```python
from build123d import *

# Parameters (mm, degrees)
SKETCH_1_W          = 1980
SKETCH_1_H          = 530
SKETCH_1_W_2        = 1920
SKETCH_1_H_2        = 470
EXTRUDE_1_DEPTH     = 30
SKETCH_2_W          = 68
SKETCH_2_H          = 30
EXTRUDE_2_DEPTH     = 68
SKETCH_3_R          = 23.5
CUT_EXTRUDE_1_DEPTH = 1125.999555555
SKETCH_4_W          = 31
SKETCH_4_H          = 470
EXTRUDE_3_DEPTH     = 30
SKETCH_5_R          = 3
CUT_EXTRUDE_2_DEPTH = 1030.528532873
SKETCH_6_R          = 3
CUT_EXTRUDE_3_DEPTH = 1030.528532873
SKETCH_7_W          = 883.399544852
SKETCH_7_H          = 30
CUT_EXTRUDE_4_DEPTH = 1125.999555555
SKETCH_8_R          = 3
CUT_EXTRUDE_5_DEPTH = 1125.999555555


with BuildPart() as part:
    # 草图1 → 凸台-拉伸1 (new body)
    with BuildSketch(Plane(origin=(0, 0, 0), x_dir=(1, 0, 0), z_dir=(0, 1, 0))):
        Rectangle(SKETCH_1_W, SKETCH_1_H)
        Rectangle(SKETCH_1_W_2, SKETCH_1_H_2, mode=Mode.SUBTRACT)
    extrude(amount=EXTRUDE_1_DEPTH)

    # 草图2 → 凸台-拉伸2 (add)
    with BuildSketch(Plane.XZ):
        with Locations((0, 250)):
            Rectangle(SKETCH_2_W, SKETCH_2_H)
        with Locations((0, -250)):
            Rectangle(SKETCH_2_W, SKETCH_2_H)
    extrude(amount=EXTRUDE_2_DEPTH)

    # 草图3 → 切除-拉伸1 (cut, through all)
    with BuildSketch(Plane.XY.offset(265)):
        with Locations((0, -30)):
            Circle(SKETCH_3_R)
    extrude(amount=-CUT_EXTRUDE_1_DEPTH, mode=Mode.SUBTRACT)

    # 草图4 → 凸台-拉伸3 (add)
    with BuildSketch(Plane(origin=(0, 30, 0), x_dir=(1, 0, 0), z_dir=(0, 1, 0))):
        with Locations((764.5, 0)):
            Rectangle(SKETCH_4_W, SKETCH_4_H)
    extrude(amount=-EXTRUDE_3_DEPTH)

    # 草图5 → 切除-拉伸2 (cut, through all)
    with BuildSketch(Plane(origin=(0, 30, 0), x_dir=(1, 0, 0), z_dir=(0, 1, 0))):
        with Locations(Location((759, 180, 0), (0, 0, 270))):
            Circle(SKETCH_5_R)
        with Locations(Location((774.5, 180, 0), (0, 0, 270))):
            Circle(SKETCH_5_R)
        with Locations(Location((759, -180, 0), (0, 0, 270))):
            Circle(SKETCH_5_R)
        with Locations(Location((774.5, -180, 0), (0, 0, 270))):
            Circle(SKETCH_5_R)
    extrude(amount=-CUT_EXTRUDE_2_DEPTH, mode=Mode.SUBTRACT)

    # 草图6 → 切除-拉伸3 (cut, symmetric)
    with BuildSketch(Plane(origin=(0, 30, 0), x_dir=(1, 0, 0), z_dir=(0, 1, 0))):
        with Locations(Location((840, -250, 0), (0, 0, 270))):
            Circle(SKETCH_6_R)
    cut_extrude_3 = extrude(amount=CUT_EXTRUDE_3_DEPTH, both=True, mode=Mode.SUBTRACT)

    # 镜向1: 切除-拉伸3 across plane
    add(cut_extrude_3.mirror(Plane.XY), mode=Mode.SUBTRACT)

    # 草图7 → 切除-拉伸4 (cut, through all)
    with BuildSketch(Plane.XY.offset(265)):
        with Locations((-591.699772426, 15)):
            Rectangle(SKETCH_7_W, SKETCH_7_H)
    extrude(amount=-CUT_EXTRUDE_4_DEPTH, mode=Mode.SUBTRACT)

    # 草图8 → 切除-拉伸5 (cut, through all)
    with BuildSketch(Plane.XY.offset(265)):
        with Locations((-100, 15)):
            Circle(SKETCH_8_R)
    extrude(amount=-CUT_EXTRUDE_5_DEPTH, mode=Mode.SUBTRACT)


solid = part.part
```
Read the model definition and answer for the solid it produces. Units are mm, in the model's axes. A direction names the side the tool comes from. Coordinates: 2 decimals unless noted, no trailing zeros. Loops run counter-clockwise (first coordinate to the right, second up) from the corner with the lowest first, then second, coordinate; pieces in that order, holes last.
(1) The mould has two halves that part along Z. Classify faces 1 (the face through (-93, 0, -250)), 2 (the face through (960, 15, 3)): released by +Z, released by -Z, zero draft, split by the parting line, or undercut.
Solution:
face 1: zero draft
face 2: undercut
(2) The part is cut by section A-A (y = -30). Determine the outline of the cut face in (x, z).
Solution:
outline: (-34, -265) - (-23.5, -265) - (-23.5, -235) - (-34, -235) - close; (-34, 235) - (-23.5, 235) - (-23.5, 265) - (-34, 265) - close; (23.5, -265) - (34, -265) - (34, -235) - (23.5, -235) - close; (23.5, 235) - (34, 235) - (34, 265) - (23.5, 265) - close
(3) Flat-ended cylindrical pins translate along their axes: pin 1 Ø24 at (y, z) = (-42.5, 249.5) entering from -X; pin 2 Ø15 at (y, z) = (15, 107.5) entering from -X; pin 3 Ø9 at (y, z) = (-43.5, -256.5) entering from +X. Find the tip coordinate at first contact, or state that the pin passes through.
Solution:
pin 1: stops at x = -34
pin 2: stops at x = 749
pin 3: stops at x = 34
(4) The part is cut by section C-C (x = 884.5). Determine the outline of the cut face in (y, z), and give its area (3 significant figures).
Solution:
outline: (0, -265) - (30, -265) - (30, -235) - (0, -235) - close; (0, 235) - (30, 235) - (30, 265) - (0, 265) - close
area: 1,800 mm2
(5) The part is cut by section B-B (z = -149.5). Determine the outline of the cut face in (x, y).
Solution:
outline: (749, 0) - (780, 0) - (780, 30) - (749, 30) - close; (960, 0) - (990, 0) - (990, 30) - (960, 30) - close
(6) A tool of negligible diameter and unlimited length cuts with its end or side. For faces 3 (the face through (869, 15, 235)), 4 (the face through (264, 6, -235)), 5 (the face through (34, -34, -250)), 6 (the face through (-93, 0, 250)), from which of +Z, -Z, +X, -X, +Y, -Y can it reach the whole face along a straight path? Write none if from no direction.
Solution:
face 3: +Y, -Y
face 4: -X, +Y, -Y
face 5: +Z, -Z, +X, -Y
face 6: +Z, -Z, -X, -Y
(7) Consider line 1 along Z through (x, y) = (774, 22); line 2 along X through (y, z) = (17, 180); line 3 along Z through (x, y) = (840, 8). Determine where each line is inside the solid, lowest interval first.
Solution:
line 1: z = -265 to -182.96, -177.04 to 177.04, 182.96 to 265
line 2: x = 749 to 756, 762 to 771.5, 777.5 to 780, 960 to 990
line 3: z = -265 to -253, -247 to -235, 235 to 247, 253 to 265
